from build123d import *

# Parameters (mm, degrees)
PAD_DEPTH   = 5
FILLET_R    = 3
FILLET001_R = 3


with BuildPart() as fillet_body:
    # Sketch → Pad (new body, symmetric)
    with BuildSketch(Plane.XZ):
        with BuildLine():
            Line((-8.074896, 40.500361), (10.74188, 40.500361))
            ThreePointArc((15.279556, 37.342338), (13.506098, 39.633148), (10.74188, 40.500361))
            Line((15.279556, 37.342338), (15.948128, 35.53762))
            ThreePointArc((13.676512, 31.587292), (15.738151, 33.030062), (15.948128, 35.53762))
            Line((13.676512, 31.587292), (7.761121, 30.557998))
            ThreePointArc((7.761121, 30.557998), (4.537487, 28.291566), (4.234332, 24.362619))
            Line((4.234332, 24.362619), (13.501884, 0))
            Line((13.501884, 0), (-6.832076, 0))
            Line((-10.03093, 38.37449), (-6.832076, 0))
            ThreePointArc((-8.074896, 40.500361), (-9.519316, 39.866568), (-10.03093, 38.37449))
        make_face()
    extrude(amount=PAD_DEPTH, both=True)

    # Fillet
    fillet_edges = [fillet_body.edges().sort_by_distance(p)[0] for p in [
        (-9.519316, -5, 39.866568),
        (1.333492, -5, 40.500361),
        (13.506098, -5, 39.633148),
        (15.613842, -5, 36.439979),
        (15.738151, -5, 33.030062),
        (10.718817, -5, 31.072645),
        (4.537487, -5, 28.291566),
        (8.868108, -5, 12.181309),
        (3.334904, -5, 0),
        (-8.431503, -5, 19.187245),
        (-9.519316, 5, 39.866568),
        (1.333492, 5, 40.500361),
        (13.506098, 5, 39.633148),
        (15.613842, 5, 36.439979),
        (15.738151, 5, 33.030062),
        (10.718817, 5, 31.072645),
        (4.537487, 5, 28.291566),
        (8.868108, 5, 12.181309),
        (3.334904, 5, 0),
        (-8.431503, 5, 19.187245),
    ]]
    fillet(fillet_edges, radius=FILLET_R)


with BuildPart() as fillet001:
    # Sketch001 → Revolution (revolve)
    with BuildSketch(Plane.XZ):
        Polygon((0, 30), (16, 0), (0, 0), align=None)
    revolve(axis=Axis((0, 0, 0), (0, 0, 1)))

    # Fusion: union Fillet body
    add(fillet_body.part)

    # Fillet001
    fillet001_edges = [fillet001.edges().sort_by_distance(p)[0] for p in [
        (-16, 0, 0),
    ]]
    fillet(fillet001_edges, radius=FILLET001_R)


solid = fillet001.part
The listing builds one solid part. Answer for the finished solid, in the listing's coordinates (mm). A direction names the side the tool comes from. Give positions to 0.01 mm unless a question says otherwise; leave off trailing zeros. Write each loop counter-clockwise with the first axis right and the second up, starting at its lowest first coordinate (ties: lowest second). Pieces come first, ordered by that corner, then holes.
1) A tool of negligible diameter and unlimited length cuts with its end or side. For faces 4 (the face through (10.76, -0.03, 31.08)), 5 (the face through (5.21, 3.75, 20.22)), 6 (the face through (5.21, -3.75, 20.22)), 7 (the face through (-8.111, -4.145, 26.206)), from which of +Z, -Z, +X, -X, +Y, -Y can it reach the whole face along a straight path? Write none if from no direction.
2) Section C-C (z = 3) is taken. Write down the section's boundary in (x, y), and give its area (3 significant figures).
3) For a pull along Z with two mould halves and no side action, classify faces 1 (the face through (10.606, 4.145, 31.969)), 2 (the face through (15.61, -0.03, 36.45)), 3 (the face through (0, 0, 0)) as pulls with the +Z half, pulls with the -Z half, needs draft (parallel to the pull), parting line crosses it, or undercut.
4) Find the intervals of material crossed by L1, parallel to Y at x = -5, z = 21.5; L2, parallel to Z at x = 5.5, y = -8.5; L3, parallel to X at y = -1.75, z = 27.5, in increasing order.
5) Section B-B (y = 0) is taken. Write down the section's boundary in (x, z).
6) Given P1, Ø10, axis at x = 2.5, z = 25, coming from the +Y side; P2, Ø2, axis at y = 5, z = 26, coming from the +X side; P3, Ø3, axis at x = -9, z = 10, coming from the -Y side, each flat-ended and moving along its own axis, determine where each tip first touches the part or whether it passes through.
7) Section A-A (x = 0) is taken. Write down the section's boundary in (y, z) (3 decimals).
Response:
1. face 4: +X, +Y, -Y
1. face 5: +X, +Y
1. face 6: +X, -Y
1. face 7: -X, -Y
2. outline: circle Ø28 at (0, 0)
2. area: 616 mm2
3. face 1: undercut
3. face 2: pulls with the +Z half
3. face 3: pulls with the -Z half
4. L1: y = -5 to 5
4. L2: z = 0 to 11.02
4. L3: x = -9.12 to 4.18
5. outline: (-13.65, 4.41) arc R3 ccw to (-11, 0) - (11, 0) arc R3 ccw to (13.65, 4.41) - (7.29, 16.33) - (4.23, 24.36) arc R4.62 cw to (7.76, 30.56) - (13.68, 31.59) arc R2.96 ccw to (15.95, 35.54) - (15.28, 37.34) arc R4.84 ccw to (10.74, 40.5) - (-8.07, 40.5) arc R1.96 ccw to (-10.03, 38.37) - (-8.07, 14.87) - close
6. P1: stops at y = 5.11
6. P2: stops at x = 3.17
6. P3: stops at y = -7.96
7. outline: (-13.647, 4.412) arc R3 ccw to (-11, 0) - (11, 0) arc R3 ccw to (13.647, 4.412) - (5, 20.625) - (5, 37.5) arc R3 ccw to (2, 40.5) - (-2, 40.5) arc R3 ccw to (-5, 37.5) - (-5, 20.625) - close
